Source: three-view drawing plus pictorial views. Frame: mm from the lowest corner of the part. Give positions to 0.01 mm unless a question says otherwise; leave off trailing zeros. Loops run counter-clockwise (first coordinate to the right, second up) from the corner with the lowest first, then second, coordinate; pieces in that order, holes last. Notation, with made-up numbers: (32, 4) - (72, 4) arc R20 ccw to (72, 16) - close; hole circle Ø3 at (21, -0.5). An arc over 180 degrees is marked (long way). Answer as a JSON object with one key per item and string values.
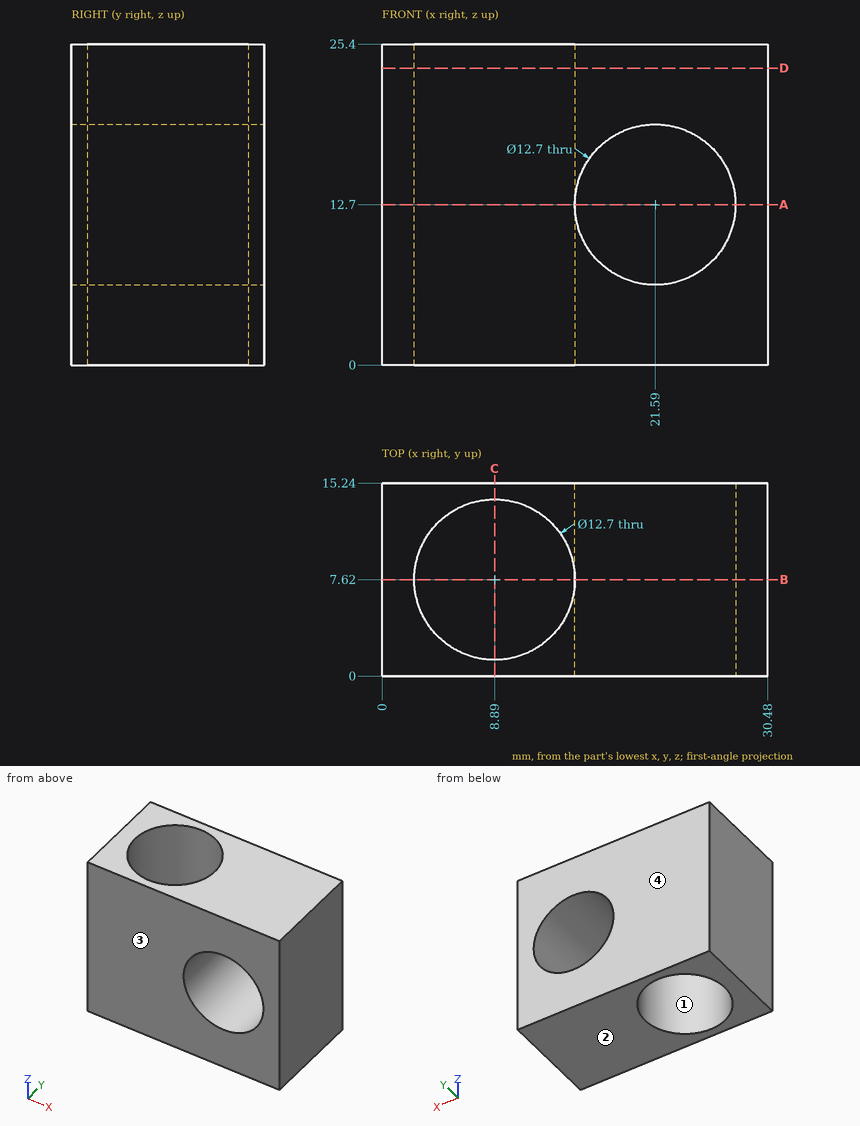
Item 1: Mould query, pull axis Y, two halves, no side actions, for the marked faces 1, 2, 3 and 4. Classes: released by +Y, released by -Y, zero draft, split by the parting line, or undercut.
Geometry check:
{"face 1": "undercut", "face 2": "zero draft", "face 3": "released by -Y", "face 4": "released by +Y"}
Item 2: Cut plane D-D (z = 23.5). Return loops of the section in (x, y).
Geometry check:
{"outline": "(0, 0) - (30.48, 0) - (30.48, 15.24) - (0, 15.24) - close; hole circle Ø12.7 at (8.89, 7.62)"}
Item 3: Cut plane A-A (z = 12.7). Return loops of the section in (x, y), then the cut area to 3 significant figures.
Geometry check:
{"outline": "(0, 0) - (15.24, 0) - (15.24, 15.24) - (0, 15.24) - close; (27.94, 0) - (30.48, 0) - (30.48, 15.24) - (27.94, 15.24) - close; hole circle Ø12.7 at (8.89, 7.62)", "area": "144 mm2"}
Item 4: Cut plane B-B (y = 7.62). Return loops of the section in (x, z), then the cut area to 3 significant figures.
Geometry check:
{"outline": "(0, 0) - (2.54, 0) - (2.54, 25.4) - (0, 25.4) - close; (15.24, 0) - (30.48, 0) - (30.48, 25.4) - (15.24, 25.4) - close; hole circle Ø12.7 at (21.59, 12.7)", "area": "325 mm2"}
Item 5: Material intervals for line 1 (X direction, y = 9.75, z = 12.7); line 2 (X direction, y = 3.25, z = 18); line 3 (Y direction, x = 8.89, z = 14.5), sorted ascending. Write a range as [from, to].
Geometry check:
{"line 1": "x = [0, 2.91], [14.87, 15.24], [27.94, 30.48]", "line 2": "x = [0, 4.28], [13.5, 18.09], [25.09, 30.48]", "line 3": "y = [0, 1.27], [13.97, 15.24]"}
Item 6: Cut plane C-C (x = 8.89). Return loops of the section in (y, z).
Geometry check:
{"outline": "(0, 0) - (1.27, 0) - (1.27, 25.4) - (0, 25.4) - close; (13.97, 0) - (15.24, 0) - (15.24, 25.4) - (13.97, 25.4) - close"}
